Verification items for the finished model (mm, model axes). A direction names the side the tool comes from. Give positions to 0.01 mm unless a question says otherwise; leave off trailing zeros. Loops run counter-clockwise (first coordinate to the right, second up) from the corner with the lowest first, then second, coordinate; pieces in that order, holes last. Notation, with made-up numbers: (35.5, 15.25) -> (40.5, 15.25) arc R17 ccw to (40.5, 28.25) -> close; hole circle Ø11 at (10, 17.5). An arc over 180 degrees is marked (long way). Answer in a Markdown table with one row per item. Add a question column.
Q1. Set-up check for faces 1 (the face through (124.352, 87, 5)), 2 (the face through (168.56, 46.06, 5.12)), 3 (the face through (33.02, 8, 5)), 4 (the face through (117.953, 76.764, 4.548)): record each of +Z, -Z, +X, -X, +Y, -Y from which the full face is reachable in a straight line by a thin tool's end or side.
Q2. Release check for a two-part mould opening along X. For faces 5 (the face through (96, 91.44, 5)), 6 (the face through (130, 9.525, 5)) record: pulls with the +X half, pulls with the -X half, needs draft (parallel to the pull), parting line crosses it, or undercut.
Q3. Section check A-A on y = 14.5. Enter the section's corners in (x, z) (1 decimal), and give its area (3 significant figures).
Q4. Gauge pin test, flat ends, axial feed: P1, Ø4, axis at y = 19.3, z = 4.76, coming from the -X side; P2, Ø5, axis at y = 5.5, z = 2.5, coming from the -X side; P3, Ø5, axis at x = 46.5, z = 5.5, coming from the +Y side; P4, Ø6, axis at x = 48.5, y = 56.5, coming from the -Z side. Record the tip position at first contact, or that the pin passes through.
Q5. Material ranges on probe 1 along X at (y, z) = (14, 2); probe 2 along Y at (x, z) = (102.5, 5.25); probe 3 along Y at (x, z) = (101, 7.75), recorded low to high.
Autodesk Inventor part; units mm, degrees
ref_plane "YZ Plane" through (0, 0, 0) normal (1, 0, 0) x (0, 1, 0)
ref_plane "XZ Plane" through (0, 0, 0) normal (0, 1, 0) x (-1, 0, 0)
ref_plane "XY Plane" through (0, 0, 0) normal (0, 0, 1) x (1, 0, 0)
sketch "Sketch1" plane through (0, 0, 0) normal (0, 0, 1) x (1, 0, 0)
  line L0 (0, 0) -> (175, 0)
  line L1 (175, 0) -> (175, 91.44)
  line L2 (175, 91.44) -> (76.7273, 91.44)
  line L3 (76.7273, 91.44) -> (0, 0)
  dimension "d0" = 175
  dimension "d1" = 91.44
  dimension "d100" = 50
extrude "Extrusion1" add sketch "Sketch1" along normal blind 9.525
sketch "Sketch8" plane through (0, 0, 0) normal (0, 0, -1) x (-1, 0, 0)
  circle A0 centre (-106.6758, 31.4833) radius 6.35
  circle A1 centre (-106.6758, 11.5887) radius 6.35
  dimension "d101" = 12.7
  dimension "d102" = 12.7
extrude "Extrusion2" cut sketch "Sketch8" against normal blind 25.4
sketch "Sketch9" plane through (0, 0, 0) normal (0, -1, 0) x (1, 0, 0)
  line L0 (175, 9.525) -> (0, 9.525)
  line L1 (0, 0) -> (0, 9.525)
  line L2 (0, 0) -> (175, 0)
  line L3 (33.02, 9.525) -> (80.01, 9.525)
  line L4 (80.01, 9.525) -> (80.01, 0)
  line L5 (80.01, 0) -> (33.02, 0)
  line L6 (33.02, 0) -> (33.02, 9.525)
  dimension "d105" = 33.02
  dimension "d106" = 46.99
extrude "Extrusion3" cut sketch "Sketch9" against normal blind 16.51 contours L4 L2 L6 L0
sketch "Sketch12" plane through (76.7273, 91.44, 0) normal (0, 1, 0) x (1, 0, 0)
  line L0 (-76.7273, -9.525) -> (0, -9.525)
  line L1 (0, 0) -> (0, -9.525)
  line L2 (0, 0) -> (-76.7273, 0)
  line L3 (-76.7273, 0) -> (-76.7273, -9.525)
  line L4 (-24.13, 0) -> (-33.655, 0)
  line L5 (-33.655, 0) -> (-33.655, -9.525)
  line L6 (-33.655, -9.525) -> (-24.13, -9.525)
  line L7 (-24.13, -9.525) -> (-24.13, 0)
  dimension "d109" = 24.13
  dimension "d110" = 9.525
extrude "Extrusion4" cut sketch "Sketch12" against normal blind 62.992 contours L5 L2 L7 L0
sketch "Sketch13" plane through (0, 0, 0) normal (0, -1, 0) x (1, 0, 0)
  line L0 (0, 0) -> (33.02, 0)
  line L1 (0, 9.525) -> (20.32, 9.525)
  line L2 (20.32, 9.525) -> (20.32, 0)
  line L3 (20.32, 0) -> (0, 0)
  line L4 (0, 0) -> (0, 9.525)
  dimension "d113" = 20.32
extrude "Extrusion5" cut sketch "Sketch13" against normal blind 2.54
sketch "Sketch14" plane through (76.7273, 91.44, 0) normal (0, 1, 0) x (1, 0, 0)
  line L0 (0, -9.525) -> (98.2727, -9.525)
  line L1 (98.2727, 0) -> (0, 0)
  line L2 (0, 0) -> (0, -9.525)
  line L3 (38.1, 0) -> (47.625, 0)
  line L4 (47.625, 0) -> (47.625, -9.525)
  line L5 (47.625, -9.525) -> (38.1, -9.525)
  line L6 (38.1, -9.525) -> (38.1, 0)
  point P0 (-76.7273, 0)
  dimension "d116" = 9.525
  dimension "d117" = 38.1
extrude "Extrusion6" cut sketch "Sketch14" against normal blind 9.525 contours L6 L1 L4 L0
sketch "Sketch15" plane through (175, 0, 0) normal (0, -1, 0) x (1, 0, 0)
  line L0 (-94.99, 0) -> (0, 0)
  line L1 (0, 0) -> (0, 9.525)
  line L2 (0, 9.525) -> (-94.99, 9.525)
  line L3 (-38.1, 9.525) -> (-47.625, 9.525)
  line L4 (-47.625, 9.525) -> (-47.625, 0)
  line L5 (-47.625, 0) -> (-38.1, 0)
  line L6 (-38.1, 0) -> (-38.1, 9.525)
  point P0 (-175, 0)
  dimension "d120" = 38.1
  dimension "d121" = 9.525
extrude "Extrusion7" cut sketch "Sketch15" against normal blind 9.525 contours L4 L2 L6 L0
sketch "Sketch16" plane through (76.7273, 81.915, 0) normal (0, 1, 0) x (1, 0, 0)
  circle A0 centre (42.8625, -4.7625) radius 2.2479
  point P0 (-76.7273, 0)
hole "Hole7" at (119.5898, 81.915, 4.7625) direction (0, -1, 0) diameter 3.302 depth 10.16 tip angle 118
sketch "Sketch17" plane through (175, 9.525, 0) normal (0, -1, 0) x (1, 0, 0)
  circle A0 centre (-42.8625, 4.7625) radius 2.2479
  point P0 (-175, 0)
hole "Hole8" at (132.1375, 9.525, 4.7625) direction (0, 1, 0) diameter 3.302 depth 12.7 tip angle 118
sketch "Sketch18" plane through (0, 16.51, 0) normal (0, -1, 0) x (1, 0, 0)
  circle A0 centre (42.5958, 4.7625) radius 2.2479
  circle A1 centre (69.2658, 4.7625) radius 2.2479
  point P0 (0, 0)
hole "Hole9" at (42.5958, 16.51, 4.7625) at (69.2658, 16.51, 4.7625) direction (0, 1, 0) diameter 3.302 depth 10.16 tip angle 118
sketch "Sketch19" plane through (0, 0, 9.525) normal (0, 0, 1) x (1, 0, 0)
  circle A0 centre (105.912, 74.168) radius 1.8034
  circle A1 centre (105.912, 56.134) radius 1.8034
  circle A2 centre (136.9, 56.134) radius 1.8034
  circle A3 centre (136.9, 74.168) radius 1.8034
  point P0 (0, 0)
hole "Hole10" at (105.912, 74.168, 9.525) at (136.9, 74.168, 9.525) at (136.9, 56.134, 9.525) at (105.912, 56.134, 9.525) direction (0, 0, -1) diameter 2.6416 end through all
sketch "Sketch20" plane through (175, 0, 0) normal (1, 0, 0) x (0, 0, -1)
  line L0 (0, 0) -> (-9.525, 0)
  point P0 (-4.7625, 69.85)
  point P1 (-4.7625, 44.45)
  point P2 (-4.7625, 19.304)
  dimension "d152" = 19.304
  dimension "d153" = 44.45
  dimension "d154" = 69.85
hole "Hole11" at (175, 69.85, 4.7625) at (175, 44.45, 4.7625) at (175, 19.304, 4.7625) direction (-1, 0, 0) diameter 3.302 depth 12.7 tip angle 118
sketch "Sketch21" plane through (43.0723, 51.3315, 0) normal (-0.7660444, 0.6427876, 0) x (0, 0, 1)
  circle A0 centre (4.7625, -32.4146) radius 2.2479
  circle A1 centre (4.7625, 19.3379) radius 2.159
  circle A2 centre (4.7625, 44.7379) radius 2.159
  point P0 (0, -67.0086)
hole "Hole12" at (71.8292, 85.6027, 4.7625) at (55.5024, 66.1452, 4.7625) at (22.2366, 26.5005, 4.7625) direction (0.7660444, -0.6427876, 0) diameter 3.302 depth 7.62 tip angle 118
sketch "Sketch22" plane through (43.0723, 51.3315, 0) normal (-0.7660444, 0.6427876, 0) x (0, 0, 1)
  circle A0 centre (4.7625, -53.0521) radius 2.159
  point P0 (0, -67.0086)
hole "Hole13" at (8.971, 10.6913, 4.7625) direction (0.7660444, -0.6427876, 0) diameter 3.302 depth 7.62 tip angle 118
sketch "Sketch23" plane through (0, 2.54, 0) normal (0, -1, 0) x (1, 0, 0)
  circle A0 centre (9.398, 3.81) radius 1.2192
  point P0 (0, 0)
hole "Hole14" at (9.398, 2.54, 3.81) direction (0, 1, 0) diameter 1.7018 depth 2.54 tip angle 118
sketch "Sketch24" plane through (175, 0, 0) normal (0, -1, 0) x (1, 0, 0)
  circle A0 centre (-1.778, 3.81) radius 1.2192
  point P0 (-175, 0)
hole "Hole15" at (173.222, 0, 3.81) direction (0, 1, 0) diameter 1.7018 depth 5.08 tip angle 118
ref_plane "Work Plane1" through (0, 0, 0) normal (1, 0, 0) x (0, 0, -1)
sketch "Sketch25" plane through (0, 0, 0) normal (1, 0, 0) x (0, 0, -1)
  circle A0 centre (-4.7625, 39.878) radius 2.159
  point P0 (0, 0)
hole "Hole16" at (0, 39.878, 4.7625) direction (1, 0, 0) diameter 3.302 depth 76.2 tip angle 118
sketch "Sketch26" plane through (0, 0, 9.525) normal (0, 0, 1) x (1, 0, 0)
  line L0 (139.44, 43.815) -> (175, 43.815)
  line L1 (175, 40.64) -> (175, 43.815)
  line L2 (139.44, 40.64) -> (175, 40.64)
  line L3 (139.44, 40.64) -> (139.44, 43.815)
  circle A0 centre (157.22, 37.9984) radius 2.4824
  point P0 (0, 0)
  dimension "d198" = 2.6416
  dimension "d199" = 4.9648
hole "Hole17" at (157.22, 37.9984, 9.525) direction (0, 0, -1) diameter 3.302 depth 4.7625 tip angle 118
sketch "Sketch27" plane through (76.7273, 91.44, 0) normal (-0.7660444, 0.6427876, 0) x (0, 0, 1)
  circle A0 centre (4.7625, -33.02) radius 1.651
  circle A1 centre (4.7625, -7.62) radius 1.651
  line L0 (0, -37.5396) -> (9.525, -37.5396)
  line L1 (9.525, -37.5396) -> (9.525, 0)
  line L2 (0, 0) -> (9.525, 0)
  line L3 (0, 0) -> (0, -37.5396)
  point P0 (0, -119.3664)
properties part number "Chassis Right3" material "Aluminum-6061"
Taken from the geometry:
| question | item | result |
|---|---|---|
| 1 | face 1 | +Z, -Z, +Y |
| 1 | face 2 | +X |
| 1 | face 3 | +Z, -Z, -Y |
| 1 | face 4 | +Y |
| 2 | face 5 | needs draft |
| 2 | face 6 | undercut |
| 3 | outline | (12.2, 0) -> (33, 0) -> (33, 9.5) -> (12.2, 9.5) -> close; (80, 0) -> (101, 0) -> (101, 9.5) -> (80, 9.5) -> close; (112.3, 0) -> (175, 0) -> (175, 9.5) -> (112.3, 9.5) -> close; hole circle Ø3.3 at (132.1, 4.8) |
| 3 | area | 987 mm² |
| 4 | P1 | stops at x = 14.52 |
| 4 | P2 | stops at x = 2.52 |
| 4 | P3 | stops at y = 28.45 |
| 4 | P4 | passes through |
| 5 | probe 1 | x = 11.75 to 33.02, 80.01 to 100.8, 112.55 to 175 |
| 5 | probe 2 | y = 0 to 6.8, 16.37 to 26.7, 36.27 to 91.44 |
| 5 | probe 3 | y = 0 to 8.74, 14.44 to 28.64, 34.33 to 91.44 |
